from build123d import *

# Parameters (mm, degrees)
F0_R     = 99.21875
F1_DEPTH = 4.953
F4_R     = 31.75
F5_DEPTH = 62.23
F3_R     = 99.21875
F6_DEPTH = 4.953
F7_R     = 22.792955
F8_DEPTH = 62.485


with BuildPart() as f1:
    # F0 (on Front) → F1 (new body)
    with BuildSketch(Plane.XZ):
        Circle(F0_R)
    extrude(amount=-F1_DEPTH)

    # F4 (on face) → F5 (join)
    with BuildSketch(Plane.XZ):
        Circle(F4_R)
    extrude(amount=-F5_DEPTH)

    # F3 (on offset) → F6 (join)
    with BuildSketch(Plane.XZ.offset(-62.484)):
        Circle(F3_R)
    extrude(amount=F6_DEPTH)

    # F7 (on face) → F8 (cut, through all)
    with BuildSketch(Plane.XZ):
        Circle(F7_R)
    extrude(amount=-F8_DEPTH, mode=Mode.SUBTRACT)


solid = f1.part
Design review of the part built by this model. Coordinates are the model's own, in mm. A direction names the side the tool comes from. Round coordinates to 2 decimals unless told otherwise and drop trailing zeros. Loops run counter-clockwise (first coordinate to the right, second up) from the corner with the lowest first, then second, coordinate; pieces in that order, holes last. Notation, with made-up numbers: (-36.5, 31) -> (-16.5, 31) arc R31 ccw to (-16.5, 68) -> close; hole circle Ø10 at (26.5, 77). An arc over 180 degrees is marked (long way). Use one line per item in the form item = value. Start each with the question number.
Q1. For pin 1 Ø12 at (x, y) = (42, 47.5) entering from +Z; pin 2 Ø4 at (y, z) = (7, 5) entering from +X; pin 3 Ø4 at (x, z) = (-68.5, -15) entering from -Y; pin 4 Ø5 at (y, z) = (11, 23.5) entering from -X, all flat-tipped, find the tip position at first contact; note any pin that passes through.
Q2. We need section C-C on y = 43. Give the boundary of the cut face in (x, z), then the cut area to 3 significant figures.
Q3. Wall thickness on line 1 along Y through (x, z) = (-44, 48.5); line 2 along Z through (x, y) = (0, 26); line 3 along X through (y, z) = (59, 2): over which ranges is each line inside the solid? List them lowest first. Write a range as [from, to].
Q4. We need section A-A on z = 0. Give the boundary of the cut face in (x, y), then the cut area to 3 significant figures.
Q5. We need section D-D on x = 0. Give the boundary of the cut face in (y, z).
Q6. We need section B-B on x = -86. Give the boundary of the cut face in (y, z), then the cut area to 3 significant figures.
Q7. Machinability: for faces 1 (the face through (-23, 4.953, 23)), 2 (the face through (-1, 62.484, 23)), which of the approach directions +Z, -Z, +X, -X, +Y, -Y give a long, thin tool a straight path to every point of the face, cutting with its end or side? Answer none if there is none.
Q8. Draft analysis for pull direction Z (two halves, no side actions). For faces 3 (the face through (-21.51, 2.44, -96.86)), 4 (the face through (-18.088, 30.805, -13.869)), 5 (the face through (-23, 57.531, 23)), state which applies: +Z half, -Z half, draft (parallel to the pull), parting line (faces both ways), or undercut.
Calculated:
q1.pin_1 = through
q1.pin_2 = 31.61
q1.pin_3 = 0
q1.pin_4 = -23.81
q2.outline = circle Ø63.5 at (0, 0); hole circle Ø45.59 at (0, 0)
q2.area = 1,530 mm²
q3.line_1 = [0, 4.95], [57.53, 62.48]
q3.line_2 = [-31.75, -22.79], [22.79, 31.75]
q3.line_3 = [-99.2, -22.71], [22.71, 99.2]
q4.outline = (-99.22, 0) -> (-22.79, 0) -> (-22.79, 62.48) -> (-99.22, 62.48) -> (-99.22, 57.53) -> (-31.75, 57.53) -> (-31.75, 4.95) -> (-99.22, 4.95) -> close; (22.79, 0) -> (99.22, 0) -> (99.22, 4.95) -> (31.75, 4.95) -> (31.75, 57.53) -> (99.22, 57.53) -> (99.22, 62.48) -> (22.79, 62.48) -> close
q4.area = 2,460 mm²
q5.outline = (0, -99.22) -> (4.95, -99.22) -> (4.95, -31.75) -> (57.53, -31.75) -> (57.53, -99.22) -> (62.48, -99.22) -> (62.48, -22.79) -> (0, -22.79) -> close; (0, 22.79) -> (62.48, 22.79) -> (62.48, 99.22) -> (57.53, 99.22) -> (57.53, 31.75) -> (4.95, 31.75) -> (4.95, 99.22) -> (0, 99.22) -> close
q6.outline = (0, -49.48) -> (4.95, -49.48) -> (4.95, 49.48) -> (0, 49.48) -> close; (57.53, -49.48) -> (62.48, -49.48) -> (62.48, 49.48) -> (57.53, 49.48) -> close
q6.area = 980 mm²
q7.face_1 = none
q7.face_2 = +Z, -Z, +X, -X, +Y
q8.face_3 = parting line
q8.face_4 = undercut
q8.face_5 = draft
